Part print with two shaded views. Sizes in mm from the minimum x, y, z corner. Give positions to 0.01 mm unless a question says otherwise; leave off trailing zeros. Write each loop counter-clockwise with the first axis right and the second up, starting at its lowest first coordinate (ties: lowest second). Pieces come first, ordered by that corner, then holes. Notation, with made-up numbers: (74.5, -37) -> (92.5, -37) arc R34 ccw to (92.5, -4) -> close; hole circle Ø4 at (50, -20). An arc over 180 degrees is marked (long way). Answer as a JSON object with one key per item and string values.
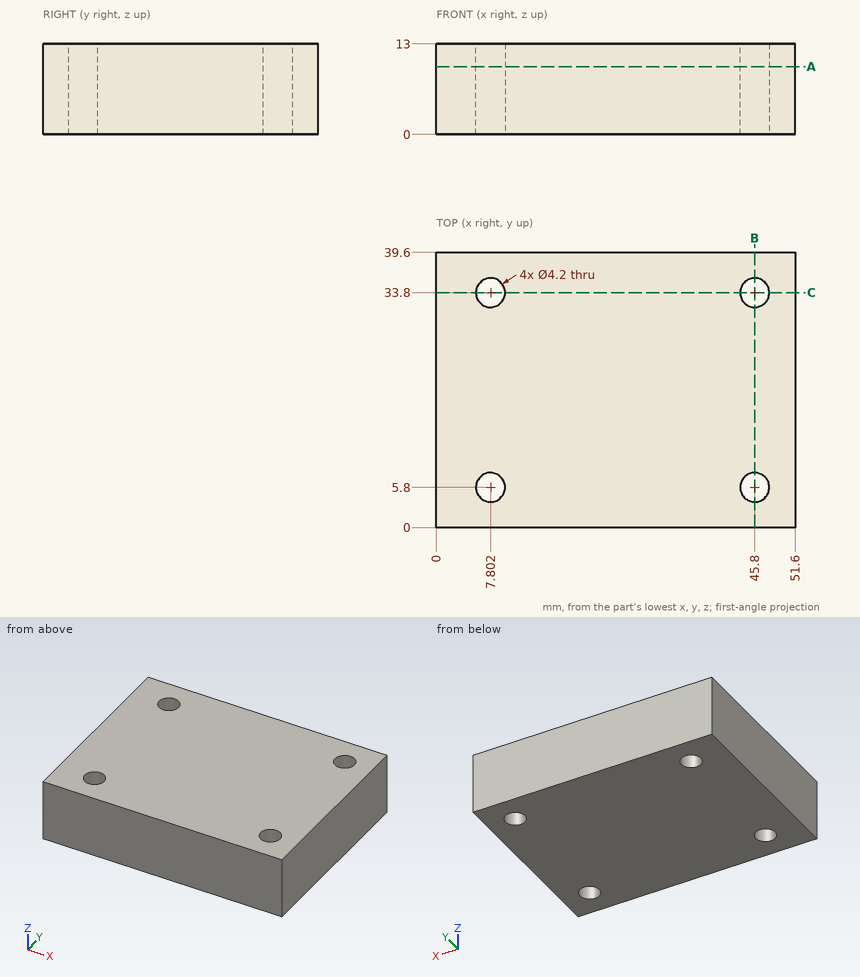
1) Pin check, flat tip, straight feed: pin 1 (5.5 mm diameter, centred on x = 45.8, y = 5.8, fed in from +Z). Stop position of the tip, or through.
Model answer:
{"pin 1": "stops at z = 13"}
2) Slice it at A-A (z = 9.75). List the corners of the cut face in (x, y), then the cut area to 3 significant figures.
Model answer:
{"outline": "(0, 0) -> (51.6, 0) -> (51.6, 39.6) -> (0, 39.6) -> close; hole circle Ø4.2 at (7.8, 5.8); hole circle Ø4.2 at (7.8, 33.8); hole circle Ø4.2 at (45.8, 5.8); hole circle Ø4.2 at (45.8, 33.8)", "area": "1,990 mm2"}
3) Slice it at C-C (y = 33.8). List the corners of the cut face in (x, z).
Model answer:
{"outline": "(0, 0) -> (5.7, 0) -> (5.7, 13) -> (0, 13) -> close; (9.9, 0) -> (43.7, 0) -> (43.7, 13) -> (9.9, 13) -> close; (47.9, 0) -> (51.6, 0) -> (51.6, 13) -> (47.9, 13) -> close"}
4) Wall check: probe 1 along Y at (x, z) = (8, 4.25); probe 2 along Y at (x, z) = (6.5, 3.75); probe 3 along X at (y, z) = (32.5, 12.75). Give the ranges that are in metal, low to high.
Model answer:
{"probe 1": "y = 0 to 3.71, 7.89 to 31.71, 35.89 to 39.6", "probe 2": "y = 0 to 4.15, 7.45 to 32.15, 35.45 to 39.6", "probe 3": "x = 0 to 6.15, 9.45 to 44.15, 47.45 to 51.6"}
5) Slice it at B-B (x = 45.8). List the corners of the cut face in (y, z).
Model answer:
{"outline": "(0, 0) -> (3.7, 0) -> (3.7, 13) -> (0, 13) -> close; (7.9, 0) -> (31.7, 0) -> (31.7, 13) -> (7.9, 13) -> close; (35.9, 0) -> (39.6, 0) -> (39.6, 13) -> (35.9, 13) -> close"}
